Work out the finished part from the listing and answer in its coordinate system (mm). Face numbers are marked on the shaded views. A direction names the side the tool comes from. Coordinates: 2 decimals unless noted, no trailing zeros. Order: outer loops, then holes, each group sorted by start corner. A loop starts at its lowest first (then second) coordinate and runs counter-clockwise, first axis right, second up. Notation, with made-up numbers: M 50,77 L 96,77 A6 ccw 96,83 Z; hole C 41.5,-38 d10. An arc over 180 degrees is marked long. Use a Markdown table: item, result.
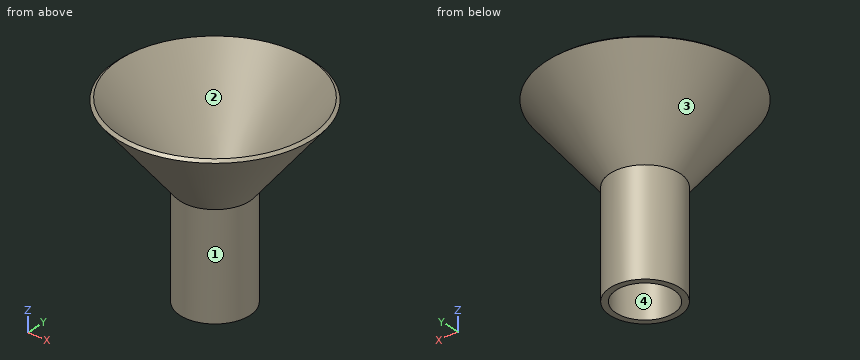
from build123d import *

# Parameters (mm, degrees)
F2_R     = 20.9909587058
F3_DEPTH = 25.4
F4_DEPTH = 25.4
F5_DEPTH = 25.4


with BuildPart() as f1:
    # F0 (on Front) → F1 (revolve)
    with BuildSketch(Plane.XZ):
        Polygon((0, -75.8221521974), (0, 0), (46.1993237782, 57.8052623537), (44.0345804445, 59.5346382788), (-3.5266100895, 0), (-25.4, 0), (-25.4, -75.8221521974), align=None)
    revolve(axis=Axis((-25.4, 0, -37.9110760987), (0, 0, 1)))

    # F2 (on face) → F3 (cut)
    with BuildSketch(Plane(origin=(0, 0, -75.8221521974), x_dir=(1, 0, 0), z_dir=(0, 0, -1))):
        with Locations((-25.4, 0)):
            Circle(F2_R)
    extrude(amount=-F3_DEPTH, mode=Mode.SUBTRACT)

    # F4 (cut): a face of the model
    f4_faces = [f1.faces().sort_by_distance(p)[0] for p in [
        (-25.4, 0, 0),
    ]]
    extrude(f4_faces, amount=-F4_DEPTH, mode=Mode.SUBTRACT)

    # F5 (cut): a face of the model
    f5_faces = [f1.faces().sort_by_distance(p)[0] for p in [
        (-25.4, 0, -25.4),
    ]]
    extrude(f5_faces, amount=-F5_DEPTH, mode=Mode.SUBTRACT)


solid = f1.part
(1) Determine the mould class of the marked faces 3 and 4 for opening direction X: pulls with the +X half, pulls with the -X half, needs draft (parallel to the pull), parting line crosses it, or undercut.
Conclusion:
| item | result |
|---|---|
| face 3 | parting line crosses it |
| face 4 | undercut |
(2) A cutting plane is placed at B-B (y = 0). Determine the outline of the cut face in (x, z).
Conclusion:
| item | result |
|---|---|
| outline | M -97,57.81 L -50.8,0 L -50.8,-75.82 L -46.39,-75.82 L -46.39,-50.8 L -47.27,-50.8 L -47.27,0 L -94.83,59.53 Z; M -4.41,-75.82 L 0,-75.82 L 0,0 L 46.2,57.81 L 44.03,59.53 L -3.53,0 L -3.53,-50.8 L -4.41,-50.8 Z |
(3) Straight lines are drawn through the part: L1, parallel to Y at x = -25.4, z = -33; L2, parallel to Y at x = -25.4, z = -68.5; L3, parallel to X at y = -4.5, z = -56.5. For each, find the intervals that lie inside material, in ascending order.
Conclusion:
| item | result |
|---|---|
| L1 | -25.4 to -21.87, 21.87 to 25.4 |
| L2 | -25.4 to -20.99, 20.99 to 25.4 |
| L3 | -50.4 to -45.9, -4.9 to -0.4 |
(4) A cutting plane is placed at A-A (x = -25.4). Determine the outline of the cut face in (y, z), then the cut area to 3 significant figures.
Conclusion:
| item | result |
|---|---|
| outline | M -71.6,57.81 L -25.4,0 L -25.4,-75.82 L -20.99,-75.82 L -20.99,-50.8 L -21.87,-50.8 L -21.87,0 L -69.43,59.53 Z; M 20.99,-75.82 L 25.4,-75.82 L 25.4,0 L 71.6,57.81 L 69.43,59.53 L 21.87,0 L 21.87,-50.8 L 20.99,-50.8 Z |
| area | 994 mm2 |
(5) A cutting plane is placed at C-C (z = -14). Determine the outline of the cut face in (x, y), then the cut area to 3 significant figures.
Conclusion:
| item | result |
|---|---|
| outline | C -25.4,0 d50.8; hole C -25.4,0 d43.75 |
| area | 524 mm2 |
(6) A cutting plane is placed at D-D (z = 2). Determine the outline of the cut face in (x, y).
Conclusion:
| item | result |
|---|---|
| outline | C -25.4,0 d54; hole C -25.4,0 d46.94 |
(7) Given P1, Ø12, axis at x = -63.5, z = 2, coming from the +Y side; P2, Ø8, axis at y = 25, z = -4, coming from the -X side; P3, Ø1.5, axis at y = 12, z = -11.5, coming from the +X side; P4, Ø12, axis at x = -48, z = 24, coming from the +Y side, each flat-ended and moving along its own axis, determine where each tip first touches the part or whether it passes through.
Conclusion:
| item | result |
|---|---|
| P1 | through |
| P2 | x = -39.69 |
| P3 | x = -2.63 |
| P4 | y = 44.63 |
(8) Which of the six approach directions +Z, -Z, +X, -X, +Y, -Y give full straight-line access (tool end or side, diameter ignored) to the marked faces 1 and 2?
Conclusion:
| item | result |
|---|---|
| face 1 | -Z |
| face 2 | +Z |
